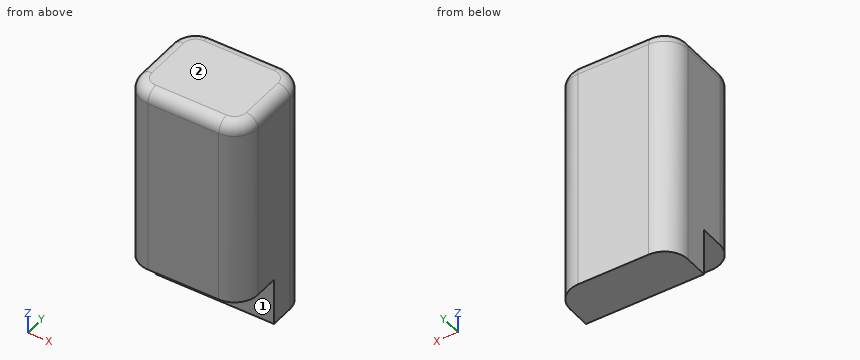
Autodesk Inventor part; units mm, degrees
ref_plane "YZ Plane" through (0, 0, 0) normal (1, 0, 0) x (0, 1, 0)
ref_plane "XZ Plane" through (0, 0, 0) normal (0, 1, 0) x (-1, 0, 0)
ref_plane "XY Plane" through (0, 0, 0) normal (0, 0, 1) x (1, 0, 0)
sketch "Sketch1" plane through (0, 0, 0) normal (0, 0, 1) x (1, 0, 0)
  line L0 (0, 0) -> (50, 0)
  line L1 (50, 0) -> (50, 20)
  line L2 (50, 20) -> (0, 20)
  line L3 (0, 20) -> (0, 0)
  dimension "d0" = 20
  dimension "d1" = 50
extrude "Extrusion1" add sketch "Sketch1" along normal blind 20
sketch "Sketch2" plane through (0, 0, 20) normal (0, 0, 1) x (1, 0, 0)
  line L0 (50, 20) -> (0, 20)
  line L1 (0, 20) -> (50, 20)
  line L2 (50, 20) -> (50, -20)
  line L3 (50, -20) -> (0, -20)
  line L4 (0, -20) -> (0, 20)
  point P0 (0, 0)
  dimension "d4" = 50
  dimension "d5" = 40
extrude "Extrusion2" add sketch "Sketch2" along normal blind 80
fillet "Fillet1" radius 10 4 edges at (50, 20, 50) (0, 20, 50) (50, -20, 60) (0, -20, 60)
fillet "Fillet2" radius 5 8 edges at (50, 0, 100) (47.0711, -17.0711, 100) (25, -20, 100) (2.9289, -17.0711, 100) (0, 0, 100) (2.9289, 17.0711, 100) (25, 20, 100) (47.0711, 17.0711, 100)
properties part number "Throttle Handler" material "Acetal Resin, Black"
The listing builds one solid part. Answer for the finished solid, in the listing's coordinates (mm). Face numbers are marked on the shaded views. A direction names the side the tool comes from. Coordinates: 2 decimals unless noted, no trailing zeros. Loops run counter-clockwise (first coordinate to the right, second up) from the corner with the lowest first, then second, coordinate; pieces in that order, holes last. Notation, with made-up numbers: M 19.5,6 L 59.5,6 A15 ccw 59.5,21 Z; hole C -1,25.25 d5. An arc over 180 degrees is marked long. Answer as CSV lines item,"result". Start each with the question number.
(1) The part is cut by section A-A (z = 44.5). Give the vertices of the cut face in (x, y), and give its area (3 significant figures).
(2) Find the intervals of material crossed by L1, parallel to Y at x = 23, z = 18; L2, parallel to Z at x = 16.5, y = -13; L3, parallel to Z at x = 19.5, y = -17.5, in increasing order. Write a range as [from, to].
(3) For the marked faces 1 and 2, determine the directions among +Z, -Z, +X, -X, +Y, -Y from which every point of the face is accessible in a straight line to the end or side of a thin tool.
(4) The part is cut by section B-B (x = 25.5). Give the vertices of the cut face in (y, z), and give its area (3 significant figures).
(5) The part is cut by section C-C (y = -7.5). Give the vertices of the cut face in (x, z), and give its area (3 significant figures).
(6) The part is cut by section D-D (z = 7). Give the vertices of the cut face in (x, y), and give its area (3 significant figures).
(7) Given pin 1 (4 mm diameter, centred on x = 37, y = -8.5, fed in from -Z); pin 2 (1.5 mm diameter, centred on x = 5, z = 22, fed in from -Y), each flat-ended and moving along its own axis, determine where each tip first touches the part or whether it passes through.
Determined:
1,outline,"M 0,-10 A10 ccw 10,-20 L 40,-20 A10 ccw 50,-10 L 50,10 A10 ccw 40,20 L 10,20 A10 ccw 0,10 Z"
1,area,"1,910 mm2"
2,L1,"[0, 20]"
2,L2,"[20, 100]"
2,L3,"[20, 99.33]"
3,face 1,"-Z, +X, -X, -Y"
3,face 2,"+Z, +X, -X, +Y, -Y"
4,outline,"M -20,20 L 0,20 L 0,0 L 20,0 L 20,95 A5 ccw 15,100 L -15,100 A5 ccw -20,95 Z"
4,area,"3,590 mm2"
5,outline,"M 0,20 L 50,20 L 50,95 A5 ccw 45,100 L 5,100 A5 ccw 0,95 Z"
5,area,"3,990 mm2"
6,outline,"M 0,0 L 50,0 L 50,10 A10 ccw 40,20 L 10,20 A10 ccw 0,10 Z"
6,area,"957 mm2"
7,pin 1,"z = 20"
7,pin 2,"y = -19.05"
